Part print with two shaded views. Sizes in mm from the minimum x, y, z corner. Give positions to 0.01 mm unless a question says otherwise; leave off trailing zeros. Write each loop counter-clockwise with the first axis right and the second up, starting at its lowest first coordinate (ties: lowest second). Pieces come first, ordered by that corner, then holes. Notation, with made-up numbers: M -6.75,-1.75 L 10.25,-1.75 A18 ccw 10.25,20.25 Z; hole C 13.25,-36 d11. An arc over 180 degrees is marked long. Return JSON: item names as keys, results as strings. Group by question number.
Q1. Band-saw the part on D-D, the plane y = 42.5. Give the cut face in (x, z).
Q2. Band-saw the part on B-B, the plane x = 30. Give the cut face in (y, z), then the cut area to 3 significant figures.
Q3. Pull direction X, two halves, no side cores. Call the marked faces 1 and 2: +X half, -X half, draft (parallel to the pull), parting line (faces both ways), or undercut.
Q4. Wall check: probe 1 along Y at (x, z) = (50, 2.15); probe 2 along Y at (x, z) = (9, 3.1); probe 3 along Y at (x, z) = (29, 3.45). Give the ranges that are in metal, low to high.
Q5. Flat gauge pins, fed straight in: pin 1 Ø1 at (x, z) = (49, 3.5) entering from -Y; pin 2 Ø0.6 at (y, z) = (47, 3.5) entering from +X. Where does each tip first touch, or does it go through?
Q6. Band-saw the part on C-C, the plane z = 1.2. Give the cut face in (x, y).
Q7. Band-saw the part on A-A, the plane y = 50. Give the cut face in (x, z).
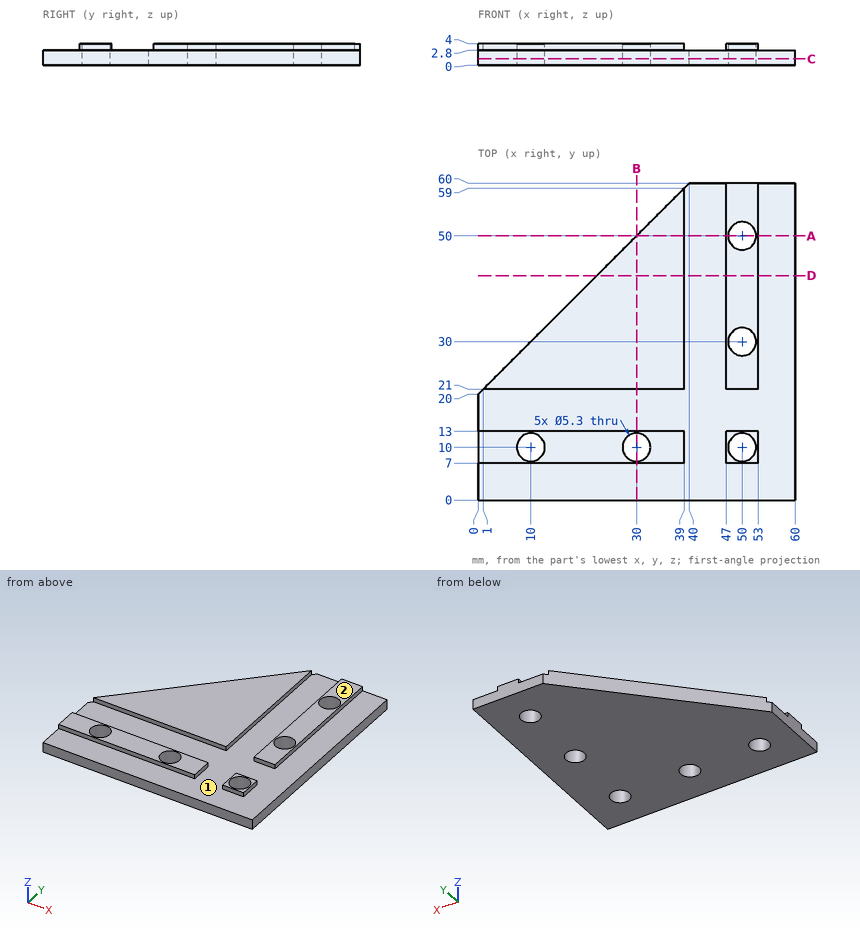
From the geometry:
{
 "1": {"outline": "M 22.5,0 L 60,0 L 60,2.8 L 53,2.8 L 53,4 L 47,4 L 47,2.8 L 39,2.8 L 39,4 L 22.5,4 Z"},
 "2": {"outline": "M 0,0 L 7.35,0 L 7.35,4 L 7,4 L 7,2.8 L 0,2.8 Z; M 12.65,0 L 50,0 L 50,4 L 21,4 L 21,2.8 L 13,2.8 L 13,4 L 12.65,4 Z", "area": "161 mm^2"},
 "3": {"face 1": "undercut", "face 2": "draft"},
 "4": {"probe 1": "y = 0 to 7.35, 12.65 to 27.35, 32.65 to 47.35, 52.65 to 60", "probe 2": "y = 7 to 7.55, 12.45 to 13, 21 to 29", "probe 3": "y = 7 to 7.55, 12.45 to 13, 21 to 49"},
 "5": {"pin 1": "stops at y = 7", "pin 2": "stops at x = 53"},
 "6": {"outline": "M 0,0 L 60,0 L 60,60 L 40,60 L 0,20 Z; hole C 10,10 d5.3; hole C 30,10 d5.3; hole C 50,10 d5.3; hole C 50,30 d5.3; hole C 50,50 d5.3"},
 "7": {"outline": "M 30,0 L 47.35,0 L 47.35,4 L 47,4 L 47,2.8 L 39,2.8 L 39,4 L 30,4 Z; M 52.65,0 L 60,0 L 60,2.8 L 53,2.8 L 53,4 L 52.65,4 Z"}
}
